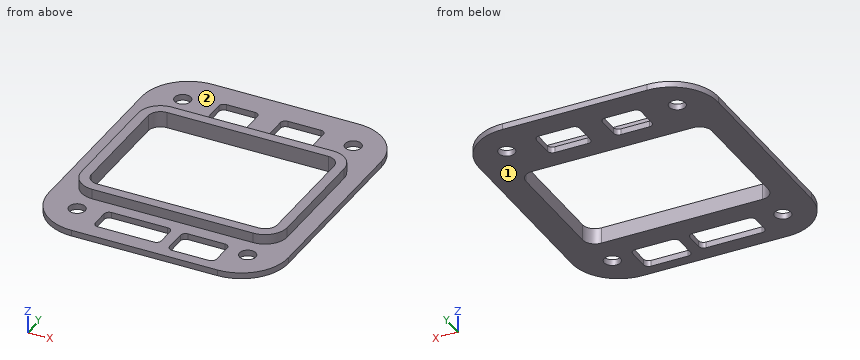
```python
from build123d import *

# Parameters (mm, degrees)
MODEL_R         = 1.62599878
EXTRUDE_1_DEPTH = 1.2
EXTRUDE_2_DEPTH = 3.2


with BuildPart() as part:
    # Model → Extrude 1 (new body)
    with BuildSketch(Plane.XY):
        with BuildLine():
            Line((91.62866358, 55.46333332), (91.62866358, 91.6983307))
            ThreePointArc((91.62866358, 91.6983307), (94.371333169, 98.448799351), (101.12180182, 101.19146894))
            Line((101.12180182, 101.19146894), (130.03882044, 101.19146894))
            ThreePointArc((130.03882044, 101.19146894), (136.765388235, 98.511299019), (139.57079782, 91.83599362))
            Line((139.57079782, 91.83599362), (139.57079782, 55.59034094))
            ThreePointArc((139.57079782, 55.59034094), (136.872269667, 48.885177471), (130.2038036, 46.09719762))
            Line((130.2038036, 46.09719762), (100.99479928, 46.09719762))
            ThreePointArc((100.99479928, 46.09719762), (94.371901783, 48.840435823), (91.62866358, 55.46333332))
        make_face()
        with Locations((98.55639928, 94.2997987)):
            Circle(MODEL_R, mode=Mode.SUBTRACT)
        with Locations((132.69399928, 53.0501987)):
            Circle(MODEL_R, mode=Mode.SUBTRACT)
        with Locations((132.69399928, 94.2997987)):
            Circle(MODEL_R, mode=Mode.SUBTRACT)
        with Locations((98.55639928, 53.0501987)):
            Circle(MODEL_R, mode=Mode.SUBTRACT)
        with BuildLine():
            Line((103.632, 50.276), (103.632, 53.6735))
            ThreePointArc((103.632, 53.6735), (103.924893219, 54.380606781), (104.632, 54.6735))
            Line((104.632, 54.6735), (115.84, 54.6735))
            ThreePointArc((115.84, 54.6735), (116.547106781, 54.380606781), (116.84, 53.6735))
            Line((116.84, 53.6735), (116.84, 50.276))
            ThreePointArc((116.84, 50.276), (116.547106781, 49.568893219), (115.84, 49.276))
            Line((115.84, 49.276), (104.632, 49.276))
            ThreePointArc((104.632, 49.276), (103.924893219, 49.568893219), (103.632, 50.276))
        make_face(mode=Mode.SUBTRACT)
        with BuildLine():
            Line((118.999, 49.26), (118.999, 53.483))
            ThreePointArc((118.999, 53.483), (119.291893219, 54.190106781), (119.999, 54.483))
            Line((119.999, 54.483), (127.397, 54.483))
            ThreePointArc((127.397, 54.483), (128.104106781, 54.190106781), (128.397, 53.483))
            Line((128.397, 53.483), (128.397, 49.26))
            ThreePointArc((128.397, 49.26), (128.104106781, 48.552893219), (127.397, 48.26))
            Line((127.397, 48.26), (119.999, 48.26))
            ThreePointArc((119.999, 48.26), (119.291893219, 48.552893219), (118.999, 49.26))
        make_face(mode=Mode.SUBTRACT)
        with BuildLine():
            Line((118.602, 96.266), (125.238, 96.266))
            ThreePointArc((125.238, 96.266), (125.945106781, 95.973106781), (126.238, 95.266))
            Line((126.238, 95.266), (126.238, 91.043))
            ThreePointArc((126.238, 91.043), (125.945106781, 90.335893219), (125.238, 90.043))
            Line((125.238, 90.043), (118.602, 90.043))
            ThreePointArc((118.602, 90.043), (117.894893219, 90.335893219), (117.602, 91.043))
            Line((117.602, 91.043), (117.602, 95.266))
            ThreePointArc((117.602, 95.266), (117.894893219, 95.973106781), (118.602, 96.266))
        make_face(mode=Mode.SUBTRACT)
        with BuildLine():
            Line((105.283, 91.043), (105.283, 95.266))
            ThreePointArc((105.283, 95.266), (105.575893219, 95.973106781), (106.283, 96.266))
            Line((106.283, 96.266), (112.03, 96.266))
            ThreePointArc((112.03, 96.266), (112.737106781, 95.973106781), (113.03, 95.266))
            Line((113.03, 95.266), (113.03, 91.043))
            ThreePointArc((113.03, 91.043), (112.737106781, 90.335893219), (112.03, 90.043))
            Line((112.03, 90.043), (106.283, 90.043))
            ThreePointArc((106.283, 90.043), (105.575893219, 90.335893219), (105.283, 91.043))
        make_face(mode=Mode.SUBTRACT)
        with BuildLine():
            Line((95.028, 61.743871815), (95.028, 83.841870988))
            ThreePointArc((95.028, 83.841870988), (96.399503395, 86.982228572), (99.58987085, 88.232997462))
            Line((99.58987085, 88.232997462), (131.847868221, 88.233000002))
            ThreePointArc((131.847868221, 88.233000002), (134.988140962, 86.861585383), (136.239, 83.671374948))
            Line((136.239, 83.671374948), (136.239, 61.573126472))
            ThreePointArc((136.239, 61.573126472), (134.867496605, 58.432768888), (131.67712915, 57.181999998))
            Line((131.67712915, 57.181999998), (99.419126585, 57.181997458))
            ThreePointArc((99.419126585, 57.181997458), (96.27876767, 58.553502055), (95.028, 61.743871815))
        make_face(mode=Mode.SUBTRACT)
    extrude(amount=EXTRUDE_1_DEPTH)

    # Model_4 → Extrude 2 (add)
    with BuildSketch(Plane.XY):
        with BuildLine():
            Line((95.028, 61.743871815), (95.028, 83.841870988))
            ThreePointArc((95.028, 83.841870988), (96.399503395, 86.982228572), (99.58987085, 88.232997462))
            Line((99.58987085, 88.232997462), (131.847868221, 88.233000002))
            ThreePointArc((131.847868221, 88.233000002), (134.988140962, 86.861585383), (136.239, 83.671374948))
            Line((136.239, 83.671374948), (136.239, 61.573126472))
            ThreePointArc((136.239, 61.573126472), (134.867496605, 58.432768888), (131.67712915, 57.181999998))
            Line((131.67712915, 57.181999998), (99.419126585, 57.181997458))
            ThreePointArc((99.419126585, 57.181997458), (96.27876767, 58.553502055), (95.028, 61.743871815))
        make_face()
        with BuildLine():
            ThreePointArc((131.699, 59.182), (133.468748117, 59.862447526), (134.239, 61.59499746))
            Line((134.239, 61.59499746), (134.239, 83.69318288))
            ThreePointArc((134.239, 83.69318288), (133.558484649, 85.46281457), (131.82599746, 86.233))
            Line((131.82599746, 86.233), (99.568, 86.23299746))
            ThreePointArc((99.568, 86.23299746), (97.798251883, 85.552549934), (97.028, 83.82))
            Line((97.028, 83.82), (97.028, 61.722))
            ThreePointArc((97.028, 61.722), (97.708446609, 59.952250241), (99.44099746, 59.18199746))
            Line((99.44099746, 59.18199746), (131.699, 59.182))
        make_face(mode=Mode.SUBTRACT)
    extrude(amount=EXTRUDE_2_DEPTH)


solid = part.part
```
For this review, take the finished solid that the model builds, in its own axes (mm). Face numbers are marked on the shaded views. A direction names the side the tool comes from. Round coordinates to 2 decimals unless told otherwise and drop trailing zeros. Write each loop counter-clockwise with the first axis right and the second up, starting at its lowest first coordinate (ties: lowest second). Pieces come first, ordered by that corner, then holes.
1) Take a section at C-C on x = 115. Give the boundary of the cut face in (y, z), then the cut area to 3 significant figures.
Answer below:
outline: (46.1, 0) - (49.28, 0) - (49.28, 1.2) - (46.1, 1.2) - close; (54.67, 0) - (59.18, 0) - (59.18, 3.2) - (57.18, 3.2) - (57.18, 1.2) - (54.67, 1.2) - close; (86.23, 0) - (101.19, 0) - (101.19, 1.2) - (88.23, 1.2) - (88.23, 3.2) - (86.23, 3.2) - close
area: 35.2 mm2
2) Take a section at B-B on y = 83. Give the boundary of the cut face in (x, z), then the cut area to 3 significant figures.
Answer below:
outline: (91.63, 0) - (97.03, 0) - (97.03, 3.2) - (95.03, 3.2) - (95.03, 1.2) - (91.63, 1.2) - close; (134.24, 0) - (139.57, 0) - (139.57, 1.2) - (136.24, 1.2) - (136.24, 3.2) - (134.24, 3.2) - close
area: 20.9 mm2
3) Insertion check: pin 1 Ø12 at (x, y) = (133.5, 94.5) entering from +Z; pin 2 Ø1 at (y, z) = (50.5, 0.5) entering from -X; pin 3 Ø1 at (y, z) = (51.5, 1) entering from +X; pin 4 Ø2.5 at (x, y) = (132.69, 94.3) entering from -Z. Each pin has a flat end and moves straight along its axis. Give the tip position at first contact, or say it passes through.
Answer below:
pin 1: stops at z = 1.2
pin 2: stops at x = 92.76
pin 3: stops at x = 138.91
pin 4: passes through
4) Take a section at D-D on z = 2.6. Give the boundary of the cut face in (x, y) (1 decimal), then the cut area to 3 significant figures.
Answer below:
outline: (95, 61.7) arc R4.5 ccw to (99.4, 57.2) - (131.7, 57.2) arc R4.5 ccw to (136.2, 61.6) - (136.2, 83.7) arc R4.5 ccw to (131.8, 88.2) - (99.6, 88.2) arc R4.5 ccw to (95, 83.8) - close; hole (97, 61.7) arc R2.5 ccw to (99.4, 59.2) - (131.7, 59.2) arc R2.5 ccw to (134.2, 61.6) - (134.2, 83.7) arc R2.5 ccw to (131.8, 86.2) - (99.6, 86.2) arc R2.5 ccw to (97, 83.8) - close
area: 261 mm2
5) For line 1 along Y through (x, z) = (109, 0.2); line 2 along X through (y, z) = (74.5, 1.25); line 3 along Y through (x, z) = (127.5, 2.85), list the stretches that pass through material, from the lowest coordinate up.
Answer below:
line 1: y = 46.1 to 49.28, 54.67 to 59.18, 86.23 to 90.04, 96.27 to 101.19
line 2: x = 95.03 to 97.03, 134.24 to 136.24
line 3: y = 57.18 to 59.18, 86.23 to 88.23
6) Take a section at A-A on x = 123.5. Give the boundary of the cut face in (y, z), then the cut area to 3 significant figures.
Answer below:
outline: (46.1, 0) - (48.26, 0) - (48.26, 1.2) - (46.1, 1.2) - close; (54.48, 0) - (59.18, 0) - (59.18, 3.2) - (57.18, 3.2) - (57.18, 1.2) - (54.48, 1.2) - close; (86.23, 0) - (90.04, 0) - (90.04, 1.2) - (88.23, 1.2) - (88.23, 3.2) - (86.23, 3.2) - close; (96.27, 0) - (101.19, 0) - (101.19, 1.2) - (96.27, 1.2) - close
area: 26.7 mm2
7) Machinability: for the marked faces 1 and 2, which of the approach directions +Z, -Z, +X, -X, +Y, -Y give a long, thin tool a straight path to every point of the face, cutting with its end or side? Answer none if there is none.
Answer below:
face 1: -Z, +X, -X, +Y, -Y
face 2: +Z
